Autodesk Inventor part; units mm, degrees
ref_plane "YZ Plane" through (0, 0, 0) normal (1, 0, 0) x (0, 1, 0)
ref_plane "XZ Plane" through (0, 0, 0) normal (0, 1, 0) x (-1, 0, 0)
ref_plane "XY Plane" through (0, 0, 0) normal (0, 0, 1) x (1, 0, 0)
sketch "Skizze1" plane through (0, 0, 0) normal (0, 0, 1) x (1, 0, 0)
  circle A0 centre (0, 0) radius 9.5
  circle A1 centre (0, 0) radius 3.05
  dimension "d0" = 6.1
  dimension "d1" = 19
extrude "Extrusion1" add sketch "Skizze1" along normal blind 2
sketch "Skizze2" plane through (0, 0, 2) normal (0, 0, 1) x (1, 0, 0)
  circle A0 centre (0, 0) radius 9.5
extrude "Extrusion2" add sketch "Skizze2" along normal blind 0.2
sketch "Skizze3" plane through (0, 0, 2.2) normal (0, 0, 1) x (1, 0, 0)
  circle A0 centre (0, 0) radius 9.5
  line L0 (0, 7.5056) -> (6.5, 3.7528)
  line L1 (6.5, 3.7528) -> (6.5, -3.7528)
  line L2 (6.5, -3.7528) -> (0, -7.5056)
  line L3 (0, -7.5056) -> (-6.5, -3.7528)
  line L4 (-6.5, -3.7528) -> (-6.5, 3.7528)
  line L5 (-6.5, 3.7528) -> (0, 7.5056)
  dimension "d6" = 13
extrude "Extrusion3" add sketch "Skizze3" along normal blind 3.5
properties part number "M8_encoderMagnet" material "ABS-Kunststoff - Schwarz"
Input: part model. Units: mm. Frame: model coordinates. A direction names the side the tool comes from. Coordinates: 2 decimals unless noted, no trailing zeros. Order: outer loops, then holes, each group sorted by start corner. A loop starts at its lowest first (then second) coordinate and runs counter-clockwise, first axis right, second up.
1. Cut plane C-C, the plane z = 1.5. Return loops of the section in (x, y), plus the area to 3 significant figures.
Checked values:
outline: circle Ø19 at (0, 0); hole circle Ø6.1 at (0, 0)
area: 254 mm2
2. Cut plane B-B, the plane y = 0. Return loops of the section in (x, z), plus the area to 3 significant figures.
Checked values:
outline: (-9.5, 0) - (-3.05, 0) - (-3.05, 2) - (3.05, 2) - (3.05, 0) - (9.5, 0) - (9.5, 5.7) - (6.5, 5.7) - (6.5, 2.2) - (-6.5, 2.2) - (-6.5, 5.7) - (-9.5, 5.7) - close
area: 50.6 mm2
3. Cut plane A-A, the plane z = 4.8. Return loops of the section in (x, y).
Checked values:
outline: circle Ø19 at (0, 0); hole (-6.5, -3.75) - (0, -7.51) - (6.5, -3.75) - (6.5, 3.75) - (0, 7.51) - (-6.5, 3.75) - close
4. Access query for faces 1 (the flat face through (6.5, 0, 4)), 2 (the flat face through (0, -4, 0)), 3 (the cylindrical face through (-3.047, -0.134, 0.986)). Directions: +Z, -Z, +X, -X, +Y, -Y. A direction counts if a zero-diameter tool reaches every point of the face in a straight line with its end or side. Return the directions, or none.
Checked values:
face 1: +Z
face 2: -Z, +X, -X, +Y, -Y
face 3: -Z
5. Contact query for flat-ended pins moving along their axis: P1, Ø3, axis at y = -4.5, z = 1, coming from the -X side; P2, Ø8, axis at x = -6, y = 3.5, coming from the +Z side; P3, Ø1, axis at x = -5.5, z = 3, coming from the -Y side; P4, Ø1.8, axis at x = -0.5, y = -0.5, coming from the -Z side. Output: stop coordinate, or through.
Checked values:
P1: stops at x = -9.01
P2: stops at z = 5.7
P3: stops at y = -8.08
P4: stops at z = 2
6. Ray query, line 1 along Y through (x, z) = (0, 1.45); line 2 along Z through (x, y) = (3, 1.5); line 3 along X through (y, z) = (2.25, 0.9). Return the intervals inside material, ascending.
Checked values:
line 1: y = -9.5 to -3.05, 3.05 to 9.5
line 2: z = 0 to 2.2
line 3: x = -9.23 to -2.06, 2.06 to 9.23
7. Cut plane D-D, the plane y = -7. Return loops of the section in (x, z).
Checked values:
outline: (-6.42, 0) - (6.42, 0) - (6.42, 5.7) - (0.88, 5.7) - (0.88, 2.2) - (-0.88, 2.2) - (-0.88, 5.7) - (-6.42, 5.7) - close
8. Draft query along X for faces 4 (the flat face through (-2.2, 6.5, 5.7)), 5 (the cylindrical face through (4.38, 8.43, 2.81)), 6 (the flat face through (-3.2, -5.66, 3.93)). Return one class per face: +X half, -X half, draft (parallel to the pull), parting line (faces both ways), or undercut.
Checked values:
face 4: draft
face 5: parting line
face 6: undercut
